```python
from build123d import *

# Parameters (mm, degrees)
F1_DEPTH = 20
F4_R     = 9.99999
F6_D     = 3
F2_W     = 4
F2_H     = 10
F7_DEPTH = 25
F8_D     = 3


# Not quite as in the source:
# - a fillet or chamfer is up to 0.001 mm smaller than in the source, because OpenCascade refuses the exact size
# - a feature names something its author has since deleted; it is built from what else it names


with BuildPart() as f1:
    # F0 (on Top) → F1 (new body)
    with BuildSketch(Plane.XY):
        with BuildLine():
            Line((0, 4), (0, 0))
            Line((0, 0), (57, 0))
            ThreePointArc((57, 0), (62.6568542495, -2.3431457505), (65, -8))
            Line((65, -8), (65, -95))
            Line((65, -95), (69, -95))
            Line((69, -95), (69, -8))
            ThreePointArc((69, -8), (65.4852813742, 0.4852813742), (57, 4))
            Line((57, 4), (0, 4))
        make_face()
    extrude(amount=F1_DEPTH)

    # F4 (radius 10 in the source; OpenCascade refuses exactly that, so slightly less here)
    f4_edges = [f1.edges().sort_by_distance(p)[0] for p in [
        (0, 2, 20),
        (0, 2, 0),
        (67, -95, 20),
        (67, -95, 0),
    ]]
    fillet(f4_edges, radius=F4_R)

    # F6 (through all)
    with Locations(Plane(origin=(65, 0, 0), x_dir=(0, -1, 0), z_dir=(-1, 0, 0))):
        with Locations((80.7573593129, 14.2426406871), (80.7573593129, 5.7573593129), (89.2426406871, 5.7573593129), (89.2426406871, 14.2426406871)):
            Hole(F6_D / 2)

    # F2 (on face) → F7 (cut)
    with BuildSketch(Plane.XZ):
        with Locations((46, 10)):
            Rectangle(F2_W, F2_H)
    extrude(amount=-F7_DEPTH, mode=Mode.SUBTRACT)

    # F8 (through all)
    with Locations(Plane.XZ):
        with Locations((8.2824855787, 3.4264645687), (21.7175144213, 16.8614934112), (20.6568542495, 4.4871247404), (9.3431457505, 15.8008332394)):
            Hole(F8_D / 2)


solid = f1.part
```
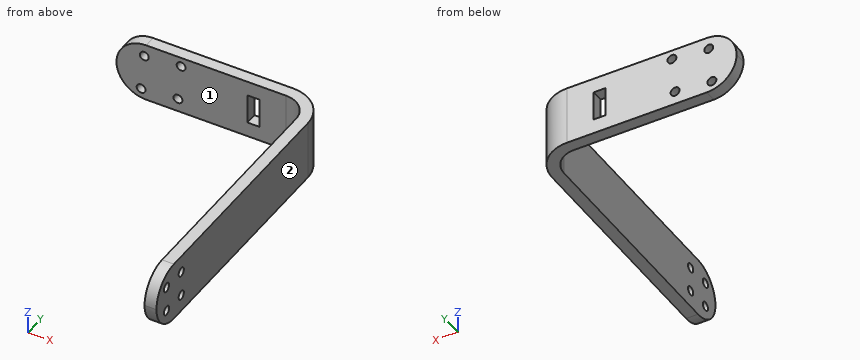
Work out the finished part from the listing and answer in its coordinate system (mm). Face numbers are marked on the shaded views. A direction names the side the tool comes from. Give positions to 0.01 mm unless a question says otherwise; leave off trailing zeros. Loops run counter-clockwise (first coordinate to the right, second up) from the corner with the lowest first, then second, coordinate; pieces in that order, holes last. Notation, with made-up numbers: (73.25, 64) -> (111.25, 64) arc R29 ccw to (111.25, 103) -> close; hole circle Ø9 at (82, -5.75). An arc over 180 degrees is marked (long way). One line per question, with ' | ' between items. Start each with the question number.
1) For the marked faces 1 and 2, determine the directions among +Z, -Z, +X, -X, +Y, -Y from which every point of the face is accessible in a straight line to the end or side of a thin tool.
2) Section A-A, the plane y = -14.5 is taken. Determine the outline of the cut face in (x, z).
3) Each of these flat-tipped pins is pushed along its axis until it touches: pin 1 (2 mm diameter, centred on x = 29, z = 12.5, fed in from -Y); pin 2 (12 mm diameter, centred on y = -24, z = 15, fed in from -X); pin 3 (4.5 mm diameter, centred on y = 1, z = 10, fed in from +X). Where does it stop, or does it pass through?
4) Section B-B, the plane x = 16.5 is taken. Determine the outline of the cut face in (y, z), then the cut area to 3 significant figures.
5) Straight lines are drawn through the part: L1, parallel to X at y = -34, z = 2.25; L2, parallel to Y at x = 34, z = 1; L3, parallel to Y at x = 59, z = 15.5. For each, find the intervals that lie inside material, in ascending order.
Resolved:
1) face 1: +Z, -Z, -X, -Y | face 2: +Z, -Z, +X, +Y, -Y
2) outline: (65, 0) -> (69, 0) -> (69, 20) -> (65, 20) -> close
3) pin 1: y = 0 | pin 2: x = 65 | pin 3: x = 66.92
4) outline: (0, 0) -> (4, 0) -> (4, 20) -> (0, 20) -> close | area: 80.0 mm2
5) L1: 65 to 69 | L2: 0 to 4 | L3: -0.25 to 3.83
